Geometry: see drawing. Coordinates: mm, zero at the bounding-box minimum. Round coordinates to 2 decimals unless told otherwise and drop trailing zeros. Loops run counter-clockwise (first coordinate to the right, second up) from the corner with the lowest first, then second, coordinate; pieces in that order, holes last. Notation, with made-up numbers: (-27.75, 83.5) - (-2.75, 83.5) arc R23 cw to (-2.75, 120.5) - close; hole circle Ø1 at (13, -24). An arc over 180 degrees is marked (long way). Use CSV: the item, a comma, the result in double quotes.
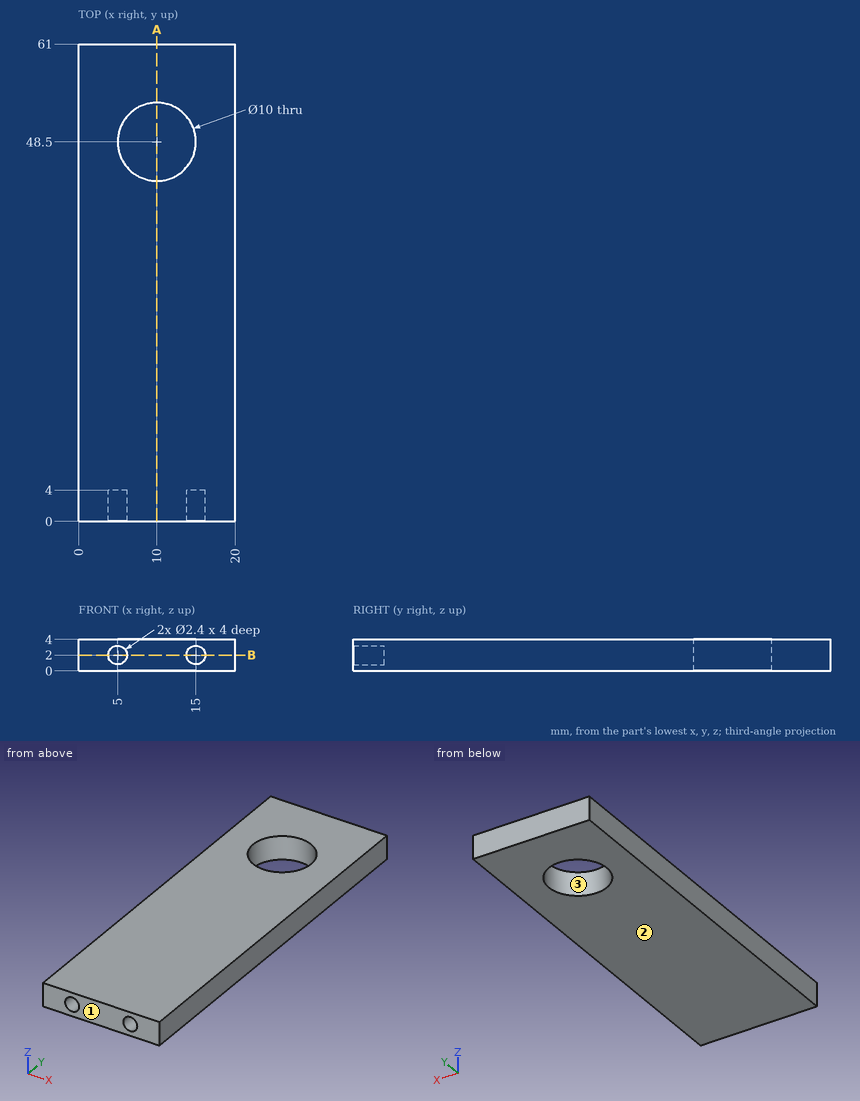
Item 1: Mould query, pull axis Y, two halves, no side actions, for the marked faces 1, 2 and 3. Classes: released by +Y, released by -Y, zero draft, split by the parting line, or undercut.
Final values:
face 1,"released by -Y"
face 2,"zero draft"
face 3,"undercut"
Item 2: Material intervals for line 1 (Z direction, x = 15, y = 1.15); line 2 (Y direction, x = 10, z = 1.1); line 3 (X direction, y = 47, z = 2.2), sorted ascending.
Final values:
line 1,"z = 0 to 0.8, 3.2 to 4"
line 2,"y = 0 to 43.5, 53.5 to 61"
line 3,"x = 0 to 5.23, 14.77 to 20"
Item 3: Pin query (flat end, axial travel): P1, Ø0.7, axis at x = 15.5, z = 2, coming from the -Y side; P2, Ø8, axis at x = 12.5, y = 50, coming from the +Z side; P3, Ø6, axis at x = 10, y = 48.5, coming from the +Z side. Return the tip coordinate at first contact, or that it passes through.
Final values:
P1,"stops at y = 4"
P2,"stops at z = 4"
P3,"passes through"
Item 4: Section B-B on z = 2. Return the cut outline in (x, y).
Final values:
outline,"(0, 0) - (3.8, 0) - (3.8, 4) - (6.2, 4) - (6.2, 0) - (13.8, 0) - (13.8, 4) - (16.2, 4) - (16.2, 0) - (20, 0) - (20, 61) - (0, 61) - close; hole circle Ø10 at (10, 48.5)"
Item 5: Section A-A on x = 10. Return the cut outline in (y, z).
Final values:
outline,"(0, 0) - (43.5, 0) - (43.5, 4) - (0, 4) - close; (53.5, 0) - (61, 0) - (61, 4) - (53.5, 4) - close"
